Check sheet for the drawn part. Datum: minimum x, y, z corner. Units: mm. A direction names the side the tool comes from. Coordinates: 2 decimals unless noted, no trailing zeros. Loops run counter-clockwise (first coordinate to the right, second up) from the corner with the lowest first, then second, coordinate; pieces in that order, holes last.
Q1. Material ranges on probe 1 along Z at (x, y) = (109.5, 20.5); probe 2 along Y at (x, z) = (52, 156); probe 3 along Y at (x, z) = (129.5, 39.5), recorded low to high.
Q2. Go/stop test with flat-tipped pins: P1, Ø6, axis at x = 47, z = 130.5, coming from the +Y side; P2, Ø11.5, axis at y = 23.5, z = 22.5, coming from the -X side; P3, Ø4, axis at x = 101.5, y = 52.5, coming from the -Z side; P4, Ø1, axis at x = 132, y = 48, coming from the +Z side. Record where each tip stops, or that it passes through.
Q3. Sectioned sample at B-B (z = 20.5). Enter the section's corners in (x, y).
Q4. Sectioned sample at C-C (y = 31). Enter the section's corners in (x, z), then the cut area to 3 significant figures.
Q5. Sectioned sample at A-A (x = 52). Enter the section's corners in (y, z).
Q6. Access from +Z, -Z, +X, -X, +Y, -Y to the whole of each face (thin tool, end or side, straight path). Record for the marked faces 1, 2 and 3.
Q7. Mould release check, pull along Z, two halves, no side actions. Record for the marked faces 4, 5 and 6: +Z half, -Z half, draft (parallel to the pull), parting line (faces both ways), or undercut.
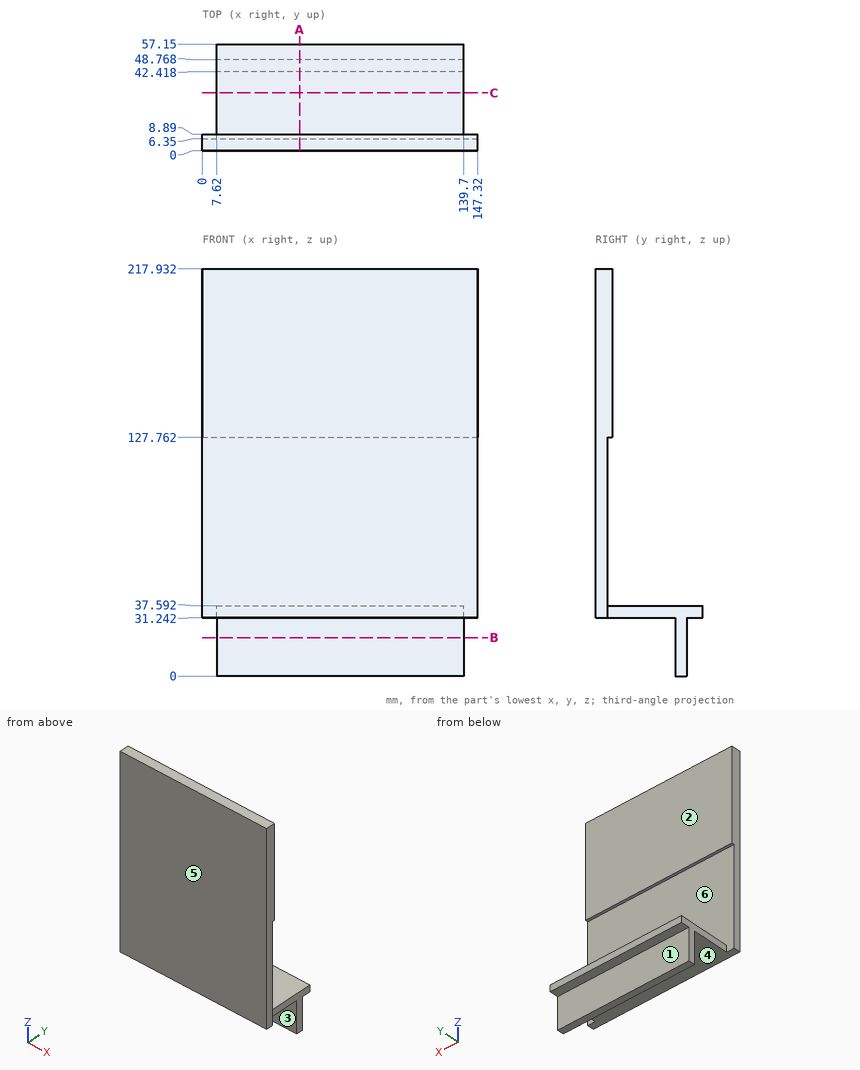
Geometry check:
1. probe 1: z = 31.24 to 37.59
1. probe 2: y = 0 to 8.89
1. probe 3: y = 0 to 6.35
2. P1: stops at y = 8.89
2. P2: passes through
2. P3: stops at z = 31.24
2. P4: stops at z = 37.59
3. outline: (7.62, 42.42) - (139.7, 42.42) - (139.7, 48.77) - (7.62, 48.77) - close
4. outline: (7.62, 31.24) - (139.7, 31.24) - (139.7, 37.59) - (7.62, 37.59) - close
4. area: 839 mm2
5. outline: (0, 31.24) - (42.42, 31.24) - (42.42, 0) - (48.77, 0) - (48.77, 31.24) - (57.15, 31.24) - (57.15, 37.59) - (6.35, 37.59) - (6.35, 127.76) - (8.89, 127.76) - (8.89, 217.93) - (0, 217.93) - close
6. face 1: -Z, +X, -X, +Y
6. face 2: +Z, +X, -X, +Y
6. face 3: -Z, +X, -X, -Y
7. face 4: -Z half
7. face 5: draft
7. face 6: undercut
